Source: CAD feature listing. Evaluate the final solid. Frame: model axes, mm. A direction names the side the tool comes from. Give positions to 0.01 mm unless a question says otherwise; leave off trailing zeros. Order: outer loops, then holes, each group sorted by start corner. A loop starts at its lowest first (then second) coordinate and runs counter-clockwise, first axis right, second up. Notation, with made-up numbers: (77.25, 67.25) -> (114.25, 67.25) arc R20 ccw to (114.25, 83.25) -> close; hole circle Ø5 at (16.5, 27). An arc over 180 degrees is marked (long way). Use CSV: the item, a comma, the result in double quotes.
Autodesk Inventor part; units mm, degrees
ref_plane "YZ Plane" through (0, 0, 0) normal (1, 0, 0) x (0, 1, 0)
ref_plane "XZ Plane" through (0, 0, 0) normal (0, 1, 0) x (-1, 0, 0)
ref_plane "XY Plane" through (0, 0, 0) normal (0, 0, 1) x (1, 0, 0)
sketch "Sketch1" plane through (0, 0, 0) normal (0, 1, 0) x (-1, 0, 0)
  line L0 (-32.55, -49.55) -> (32.55, -49.55)
  line L1 (32.55, -49.55) -> (32.55, 49.55)
  line L2 (32.55, 49.55) -> (-32.55, 49.55)
  line L3 (-32.55, 49.55) -> (-32.55, -49.55)
  line L4 (-32.55, -49.55) -> (32.55, 49.55) construction
  line L5 (32.55, -49.55) -> (-32.55, 49.55) construction
  point P0 (0, 0)
  dimension "d0" = 65.1
  dimension "d1" = 99.1
extrude "Extrusion1" add sketch "Sketch1" along normal blind 5.08
sketch "Sketch2" plane through (0, 5.08, 0) normal (0, 1, 0) x (1, 0, 0)
  line L0 (28.75, 45.75) -> (-28.75, 45.75)
  line L1 (-28.75, 45.75) -> (-28.75, -45.75)
  line L2 (-28.75, -45.75) -> (28.75, -45.75)
  line L3 (28.75, -45.75) -> (28.75, 45.75)
  line L4 (28.75, 45.75) -> (-28.75, -45.75) construction
  line L5 (-28.75, 45.75) -> (28.75, -45.75) construction
  line L6 (-32.55, 49.55) -> (-32.55, -49.55)
  line L7 (-32.55, -49.55) -> (32.55, -49.55)
  line L8 (32.55, 49.55) -> (-32.55, 49.55)
  line L9 (32.55, -49.55) -> (32.55, 49.55)
  line L10 (24.95, -41.95) -> (32.55, -49.55) construction
  line L11 (23.0931, -45.75) -> (29.7216, -52.3784)
  line L12 (35.3784, -46.7216) -> (28.75, -40.0931)
  arc A0 (29.7216, -52.3784) -> (35.3784, -46.7216) centre (32.55, -49.55) ccw
  circle A1 centre (32.55, -49.55) radius 1.375
  point P0 (0, 0)
  dimension "d4" = 3.8
  dimension "d5" = 3.8
  dimension "d22" = 8
  dimension "d23" = 2.75
extrude "Extrusion2" add sketch "Sketch2" along normal blind 48 contours L0 L1 L2 L11 L7 L6 L8 L9 L12 L3 | L12 L9 A1 L7 L11 L2 L3 | L9 L7 A1 picked at (32.448, -48.6448)
sketch "Sketch3" plane through (0, 5.08, 0) normal (0, 1, 0) x (1, 0, 0)
  line L0 (28.75, -45.75) -> (-28.75, -45.75) construction
  line L1 (0, -45.75) -> (0, 45.75) construction
  line L2 (28.75, 45.75) -> (-28.75, 45.75) construction
  circle A0 centre (-24.5, -35.75) radius 3.5
  circle A1 centre (-24.5, -35.75) radius 1.375
  line L3 (28.75, 45.75) -> (28.75, -45.75) construction
  line L4 (28.75, 0) -> (-28.75, 0) construction
  line L5 (-28.75, -45.75) -> (-28.75, 45.75) construction
  circle A2 centre (-24.5, 22.25) radius 3.5
  circle A3 centre (-24.5, 22.25) radius 1.375
  circle A4 centre (24.5, -35.75) radius 3.5
  circle A5 centre (24.5, -35.75) radius 1.375
  circle A6 centre (24.5, 22.25) radius 3.5
  circle A7 centre (24.5, 22.25) radius 1.375
  point P0 (0, 0)
  dimension "d8" = 7
  dimension "d9" = 2.75
  dimension "d10" = 10
  dimension "d11" = 24.5
  dimension "d14" = 58
extrude "Extrusion3" add sketch "Sketch3" along normal blind 5
sketch "Sketch4" plane through (0, 0, 0) normal (0, -1, 0) x (1, 0, 0)
  line L0 (31.0438, 48.2342) -> (34.0562, 50.8658) construction
  line L1 (32.55, 49.55) -> (32.55, -49.55)
  line L2 (32.55, 44.2386) -> (36.6878, 47.8534)
  line L3 (31.4245, 53.8782) -> (28.4122, 51.2466)
  arc A0 (28.4122, 51.2466) -> (27.2664, 49.55) centre (31.0438, 48.2342) ccw
  arc A1 (36.6878, 47.8534) -> (31.4245, 53.8782) centre (34.0562, 50.8658) ccw
  line L4 (-32.55, 49.55) -> (32.55, 49.55)
  line L5 (27.2664, 49.55) -> (32.55, 49.55)
  line L6 (32.55, 49.55) -> (32.55, 44.2386)
  circle A2 centre (34.0562, 50.8658) radius 1.375
  line L7 (0, 49.55) -> (0, -49.55) construction
  line L8 (32.55, -49.55) -> (-32.55, -49.55) construction
  line L9 (32.55, 0) -> (-33.3, 0) construction
  line L10 (32.55, -49.55) -> (32.55, 49.55)
  line L11 (32.55, -44.2386) -> (36.6878, -47.8534)
  line L12 (31.4245, -53.8782) -> (28.4122, -51.2466)
  arc A3 (27.2664, -49.55) -> (28.4122, -51.2466) centre (31.0438, -48.2342) ccw
  arc A4 (31.4245, -53.8782) -> (36.6878, -47.8534) centre (34.0562, -50.8658) ccw
  line L13 (-32.55, -49.55) -> (32.55, -49.55)
  circle A5 centre (34.0562, -50.8658) radius 1.375
  line L14 (-32.55, 49.55) -> (-32.55, -49.55)
  line L15 (-32.55, 44.2386) -> (-36.6878, 47.8534)
  line L16 (-31.4245, 53.8782) -> (-28.4122, 51.2466)
  arc A6 (-27.2664, 49.55) -> (-28.4122, 51.2466) centre (-31.0438, 48.2342) ccw
  arc A7 (-31.4245, 53.8782) -> (-36.6878, 47.8534) centre (-34.0562, 50.8658) ccw
  line L17 (-27.2664, 49.55) -> (-32.55, 49.55)
  circle A8 centre (-34.0562, 50.8658) radius 1.375
  arc A9 (-36.6878, -47.8534) -> (-31.4245, -53.8782) centre (-34.0562, -50.8658) ccw
  line L18 (-32.55, -44.2386) -> (-36.6878, -47.8534)
  line L19 (-31.4245, -53.8782) -> (-28.4122, -51.2466)
  arc A10 (-28.4122, -51.2466) -> (-27.2664, -49.55) centre (-31.0438, -48.2342) ccw
  circle A11 centre (-34.0562, -50.8658) radius 1.375
  line L20 (-27.2664, -49.55) -> (-32.55, -49.55)
  line L21 (-32.55, -49.55) -> (-32.55, 49.55)
  point P0 (0, 0)
  point P1 (-27.2664, -49.55)
  point P2 (-27.2664, 49.55)
  point P3 (32.55, -44.2386)
  point P4 (32.55, -49.55)
  dimension "d24" = 2
  dimension "d25" = 8
  dimension "d26" = 131.141
  dimension "d27" = 2.75
extrude "Extrusion4" add sketch "Sketch4" against normal up to surface (53.08 mm away) contours L4 A0 L3 A1 L2 L1 | L11 A4 L12 A3 L13 L1 | L4 L14 L15 A7 L16 A6 | A10 L19 A9 L18 L14 L13
fillet "Fillet2" radius 3 4 edges at (28.75, 29.08, -45.75) (-28.75, 29.08, -45.75) (-28.75, 29.08, 45.75) (28.75, 29.08, 45.75)
sketch "Sketch5" plane through (0, 5.08, 0) normal (0, 1, 0) x (1, 0, 0)
  line L0 (15, 0) -> (-15, 0) construction
  line L1 (15, 2.5) -> (-15, 2.5)
  line L2 (-15, -2.5) -> (15, -2.5)
  arc A0 (15, -2.5) -> (15, 2.5) centre (15, 0) ccw
  arc A1 (-15, 2.5) -> (-15, -2.5) centre (-15, 0) ccw
  line L3 (-25.75, -45.75) -> (25.75, -45.75) construction
  line L4 (0, -45.75) -> (0, 45.75) construction
  line L5 (-25.75, 45.75) -> (25.75, 45.75) construction
  arc A2 (-15, 12.5) -> (-15, 7.5) centre (-15, 10) ccw
  line L6 (15, 12.5) -> (-15, 12.5)
  line L7 (-15, 7.5) -> (15, 7.5)
  arc A3 (15, 7.5) -> (15, 12.5) centre (15, 10) ccw
  arc A4 (-15, 22.5) -> (-15, 17.5) centre (-15, 20) ccw
  line L8 (15, 22.5) -> (-15, 22.5)
  line L9 (-15, 17.5) -> (15, 17.5)
  arc A5 (15, 17.5) -> (15, 22.5) centre (15, 20) ccw
  arc A6 (-15, 32.5) -> (-15, 27.5) centre (-15, 30) ccw
  line L10 (15, 32.5) -> (-15, 32.5)
  line L11 (-15, 27.5) -> (15, 27.5)
  arc A7 (15, 27.5) -> (15, 32.5) centre (15, 30) ccw
  arc A8 (-15, -7.5) -> (-15, -12.5) centre (-15, -10) ccw
  line L12 (-15, -12.5) -> (15, -12.5)
  line L13 (15, -7.5) -> (-15, -7.5)
  arc A9 (15, -12.5) -> (15, -7.5) centre (15, -10) ccw
  arc A10 (-15, -17.5) -> (-15, -22.5) centre (-15, -20) ccw
  line L14 (-15, -22.5) -> (15, -22.5)
  line L15 (15, -17.5) -> (-15, -17.5)
  arc A11 (15, -22.5) -> (15, -17.5) centre (15, -20) ccw
  arc A12 (-15, -27.5) -> (-15, -32.5) centre (-15, -30) ccw
  line L16 (-15, -32.5) -> (15, -32.5)
  line L17 (15, -27.5) -> (-15, -27.5)
  arc A13 (15, -32.5) -> (15, -27.5) centre (15, -30) ccw
  point P0 (0, 0)
  dimension "d31" = 15
  dimension "d32" = 5
  dimension "d35" = 10
  dimension "d42" = 10
extrude "Extrusion5" cut sketch "Sketch5" against normal up to surface (5.08 mm away)
sketch "Sketch9" plane through (27.2664, 0, -49.55) normal (0, 0, -1) x (-1, 0, 0)
  line L0 (6.2664, 10.08) -> (-0.7336, 10.08)
  line L1 (1.3914, 10.08) -> (4.1414, 10.08)
  line L2 (1.3914, 10.08) -> (4.1414, 10.08) construction
  line L3 (2.7664, 10.08) -> (-0.7336, 10.08) construction
  line L4 (6.2664, 10.08) -> (-0.7336, 10.08)
  line L5 (0, 53.08) -> (0, 0)
  line L6 (-0.7336, 10.08) -> (0, 13.5023) construction
  line L7 (17.725, 11.35) -> (1.475, 11.35)
  line L8 (1.475, 11.35) -> (1.475, 25.6)
  line L9 (1.475, 25.6) -> (17.725, 25.6)
  line L10 (17.725, 25.6) -> (17.725, 11.35)
  line L11 (9.6, 25.6) -> (9.6, 11.35) construction
  line L12 (20.5, 11.35) -> (36.5, 11.35)
  line L13 (36.5, 11.35) -> (36.5, 27.85)
  line L14 (36.5, 27.85) -> (20.5, 27.85)
  line L15 (20.5, 27.85) -> (20.5, 11.35)
  line L16 (28.5, 27.85) -> (28.5, 11.35) construction
  line L17 (54.5, 27.85) -> (38.5, 27.85)
  line L18 (54.5, 11.35) -> (54.5, 27.85)
  line L19 (38.5, 11.35) -> (54.5, 11.35)
  line L20 (38.5, 27.85) -> (38.5, 11.35)
  point P0 (27.2664, 0)
  point P1 (46.5, 27.85)
  point P2 (46.5, 11.35)
  dimension "d58" = 3.5
  dimension "d60" = 3.5
  dimension "d63" = 16.25
  dimension "d64" = 14.25
  dimension "d65" = 1.27
  dimension "d66" = 9.6
  dimension "d69" = 16
  dimension "d70" = 16.5
  dimension "d71" = 1.27
  dimension "d72" = 28.5
  dimension "d75" = 18
extrude "Extrusion7" cut sketch "Sketch9" against normal up to surface (3.8 mm away)
properties part number "Case RevC" material "ABS Plastic"
1. Pin query (flat end, axial travel): P1, Ø2, axis at x = -24.5, z = 35.75, coming from the -Y side; P2, Ø6, axis at x = 7.5, y = 40.5, coming from the +Z side; P3, Ø1, axis at y = 43, z = 29, coming from the -X side; P4, Ø4, axis at y = 20.5, z = -47.5, coming from the -X side. Return the tip coordinate at first contact, or that it passes through.
Answer below:
P1,"stops at y = 0"
P2,"stops at z = 49.55"
P3,"stops at x = -32.55"
P4,"stops at x = -37.82"
2. Mould query, pull axis X, two halves, no side actions, for faces 5 (the flat face through (0, 34, -45.75)), 6 (the flat face through (-34.59, 26.17, 46.02)). Classes: released by +X, released by -X, zero draft, split by the parting line, or undercut.
Answer below:
face 5,"undercut"
face 6,"released by -X"
3. Access query for faces 1 (the cylindrical face through (-17.5, 2.6, 9.9)), 2 (the flat face through (24.5, 10.08, -20.7)), 3 (the flat face through (25.791, 18, -48)), 4 (the flat face through (29.94, 26.17, 52.58)). Directions: +Z, -Z, +X, -X, +Y, -Y. A direction counts if a zero-diameter tool reaches every point of the face in a straight line with its end or side. Return the directions, or none.
Answer below:
face 1,"+Y, -Y"
face 2,"+Y"
face 3,"-Z"
face 4,"+Z, +Y, -Y"
4. Section query B-B on z = 20. Return loops of the section in (x, y), plus the area to 3 significant figures.
Answer below:
outline,"(-32.55, 0) -> (-17.5, 0) -> (-17.5, 5.08) -> (-28.75, 5.08) -> (-28.75, 53.08) -> (-32.55, 53.08) -> close; (17.5, 0) -> (32.55, 0) -> (32.55, 53.08) -> (28.75, 53.08) -> (28.75, 5.08) -> (17.5, 5.08) -> close"
area,"518 mm²"
5. Section query A-A on x = 24.5. Return loops of the section in (y, z) (3 decimals).
Answer below:
outline,"(0, -49.55) -> (11.35, -49.55) -> (11.35, -45.75) -> (5.08, -45.75) -> (5.08, -25.75) -> (10.08, -25.75) -> (10.08, -23.625) -> (5.08, -23.625) -> (5.08, -20.875) -> (10.08, -20.875) -> (10.08, -18.75) -> (5.08, -18.75) -> (5.08, 32.25) -> (10.08, 32.25) -> (10.08, 34.375) -> (5.08, 34.375) -> (5.08, 37.125) -> (10.08, 37.125) -> (10.08, 39.25) -> (5.08, 39.25) -> (5.08, 45.75) -> (53.08, 45.75) -> (53.08, 49.55) -> (0, 49.55) -> close; (25.6, -49.55) -> (53.08, -49.55) -> (53.08, -45.75) -> (25.6, -45.75) -> close"
6. Section query C-C on z = -15. Return loops of the section in (x, y).
Answer below:
outline,"(-32.55, 0) -> (32.55, 0) -> (32.55, 53.08) -> (28.75, 53.08) -> (28.75, 5.08) -> (-28.75, 5.08) -> (-28.75, 53.08) -> (-32.55, 53.08) -> close"
7. Section query D-D on x = -24.5. Return loops of the section in (y, z) (3 decimals).
Answer below:
outline,"(0, -49.55) -> (11.35, -49.55) -> (11.35, -45.75) -> (5.08, -45.75) -> (5.08, -25.75) -> (10.08, -25.75) -> (10.08, -23.625) -> (5.08, -23.625) -> (5.08, -20.875) -> (10.08, -20.875) -> (10.08, -18.75) -> (5.08, -18.75) -> (5.08, 32.25) -> (10.08, 32.25) -> (10.08, 34.375) -> (5.08, 34.375) -> (5.08, 37.125) -> (10.08, 37.125) -> (10.08, 39.25) -> (5.08, 39.25) -> (5.08, 45.75) -> (53.08, 45.75) -> (53.08, 49.55) -> (0, 49.55) -> close; (27.85, -49.55) -> (53.08, -49.55) -> (53.08, -45.75) -> (27.85, -45.75) -> close"
8. Ray query, line 1 along Z through (x, y) = (-24.5, 8.5) (3 decimals); line 2 along X through (y, z) = (8.7, 35.75) (3 decimals); line 3 along Z through (x, y) = (-17, 35). Return the intervals inside material, ascending.
Answer below:
line 1,"z = -49.55 to -45.75, -25.75 to -23.625, -20.875 to -18.75, 32.25 to 34.375, 37.125 to 39.25, 45.75 to 49.55"
line 2,"x = -32.55 to -28.75, -28 to -25.875, -23.125 to -21, 21 to 23.125, 25.875 to 28, 28.75 to 32.55"
line 3,"z = -49.55 to -45.75, 45.75 to 49.55"
